CAD build for the part. Positions are in the model's coordinates, mm. A direction names the side the tool comes from. Give positions to 0.01 mm unless a question says otherwise; leave off trailing zeros. Write each loop counter-clockwise with the first axis right and the second up, starting at its lowest first coordinate (ties: lowest second). Pieces come first, ordered by that corner, then holes. Notation, with made-up numbers: (79, -5.75) - (93, -5.75) arc R22 cw to (93, 3.25) - close; hole circle Ø3 at (77, -19). An arc over 180 degrees is marked (long way). Answer as a JSON object with one key per item and string values.
from build123d import *

# Parameters (mm, degrees)
F1_DEPTH = 101.6
F2_R     = 2.38125
F3_DEPTH = 6.35
F4_R     = 5.715
F5_DEPTH = 4.064


with BuildPart() as f1:
    # F0 (on Right) → F1 (new body)
    with BuildSketch(Plane.YZ):
        Polygon((0, -31.19104), (0, -15.31604), (-2.9972, -15.31604), (-2.9972, -55.95604), (3.3528, -55.95604), (3.3528, -31.19104), align=None)
    extrude(amount=F1_DEPTH)

    # F2 (on face) → F3 (cut, through all)
    with BuildSketch(Plane(origin=(0, 3.3528, 0), x_dir=(-1, 0, 0), z_dir=(0, 1, 0))):
        with Locations((-76.552249, -43.57354)):
            Circle(F2_R)
        with Locations((-25.047751, -43.57354)):
            Circle(F2_R)
    extrude(amount=-F3_DEPTH, mode=Mode.SUBTRACT)

    # F4 (on face) → F5 (cut)
    with BuildSketch(Plane.XZ.offset(2.9972)):
        with Locations((25.047751, -43.57354)):
            Circle(F4_R)
        with Locations((76.552249, -43.57354)):
            Circle(F4_R)
    extrude(amount=-F5_DEPTH, mode=Mode.SUBTRACT)


solid = f1.part
(1) Saw through at B-B, the plane x = 47. Give the cut face in (y, z), and give its area (3 significant figures).
Answer key:
{"outline": "(-3, -55.96) - (3.35, -55.96) - (3.35, -31.19) - (0, -31.19) - (0, -15.32) - (-3, -15.32) - close", "area": "205 mm²"}
(2) Probe L1, parallel to X at y = -1, z = -48; L2, parallel to X at y = 0.5, z = -40.5; L3, parallel to Y at x = 34.5, z = -20. List the from-to ranges inside material, lowest first. Write a range as [from, to].
Answer key:
{"L1": "x = [0, 21.43], [28.66, 72.94], [80.17, 101.6]", "L2": "x = [0, 20.23], [29.87, 71.73], [81.37, 101.6]", "L3": "y = [-3, 0]"}
(3) 3-axis set-ups, long thin cutter, end or side, ignore diameter. For faces 1 (the face through (27.685, -0.994, -48.644)), 2 (the face through (50, 0, -23)), 3 (the face through (25.358, 2.226, -41.213)): which of +Z, -Z, +X, -X, +Y, -Y reach the whole face in a straight line?
Answer key:
{"face 1": "-Y", "face 2": "+Z, +X, -X, +Y", "face 3": "+Y, -Y"}
(4) Pull direction X, two halves, no side cores. Call faces 4 (the face through (75.272, 2.226, -41.566)), 5 (the face through (28, 1.067, -43)), 6 (the face through (0, -1, -40)), 7 (the face through (50, 3.353, -44)): pulls with the +X half, pulls with the -X half, needs draft (parallel to the pull), parting line crosses it, or undercut.
Answer key:
{"face 4": "undercut", "face 5": "undercut", "face 6": "pulls with the -X half", "face 7": "needs draft"}
(5) Saw through at C-C, the plane z = -39.5. Give the cut face in (x, y).
Answer key:
{"outline": "(0, -3) - (21.04, -3) - (21.04, 1.07) - (29.06, 1.07) - (29.06, -3) - (72.54, -3) - (72.54, 1.07) - (80.56, 1.07) - (80.56, -3) - (101.6, -3) - (101.6, 3.35) - (0, 3.35) - close"}
(6) Saw through at D-D, the plane z = -28. Give the cut face in (x, y).
Answer key:
{"outline": "(0, -3) - (101.6, -3) - (101.6, 0) - (0, 0) - close"}
(7) Flat gauge pins, fed straight in: P1, Ø1, axis at y = 1.5, z = -49, coming from the -X side; P2, Ø3.5, axis at x = 77, z = -43, coming from the -Y side; P3, Ø5, axis at x = 58.5, z = -26, coming from the +Y side. Where does each tip first touch, or does it go through?
Answer key:
{"P1": "stops at x = 0", "P2": "stops at y = 1.07", "P3": "stops at y = 0"}
(8) Saw through at A-A, the plane x = 24.5. Give the cut face in (y, z), and give its area (3 significant figures).
Answer key:
{"outline": "(-3, -55.96) - (3.35, -55.96) - (3.35, -45.89) - (1.07, -45.89) - (1.07, -49.26) - (-3, -49.26) - close; (-3, -37.88) - (1.07, -37.88) - (1.07, -41.26) - (3.35, -41.26) - (3.35, -31.19) - (0, -31.19) - (0, -15.32) - (-3, -15.32) - close", "area": "148 mm²"}
